Check sheet for the drawn part. Datum: minimum x, y, z corner. Units: mm. A direction names the side the tool comes from. Coordinates: 2 decimals unless noted, no trailing zeros. Loops run counter-clockwise (first coordinate to the right, second up) from the corner with the lowest first, then second, coordinate; pieces in that order, holes last.
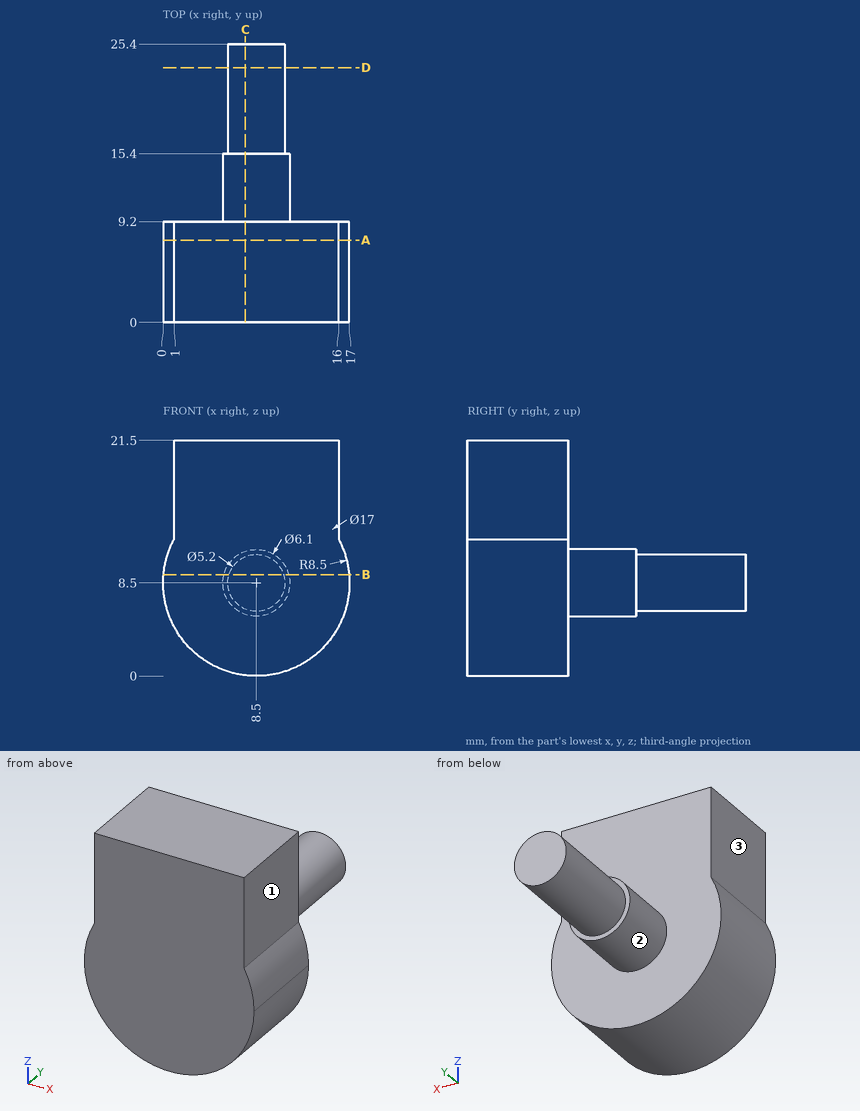
1) Scan lines: line 1 (X direction, y = 5.75, z = 16.75); line 2 (Y direction, x = 12, z = 16); line 3 (Z direction, x = 8.5, y = 11.75). Record each from-to range of solid material in increasing order.
Answer sheet:
line 1: x = 1 to 16
line 2: y = 0 to 9.2
line 3: z = 5.45 to 11.55
2) Depth check by flat-ended pin: pin 1 (4 mm diameter, centred on x = 9, y = 14.5, fed in from -Z); pin 2 (7 mm diameter, centred on y = 4, z = 16.5, fed in from +X); pin 3 (3 mm diameter, centred on y = 8, z = 15, fed in from -X); pin 4 (1 mm diameter, centred on y = 11.5, z = 19, fed in from +X). Enter the tip coordinate at first touch or a pass-through.
Answer sheet:
pin 1: stops at z = 5.45
pin 2: stops at x = 16
pin 3: stops at x = 1
pin 4: passes through
3) Section check D-D on y = 23.25. Enter the section's corners in (x, z), plus the area to 3 significant figures.
Answer sheet:
outline: circle Ø5.2 at (8.5, 8.5)
area: 21.2 mm2
4) Section check B-B on z = 9.25. Enter the section's corners in (x, y).
Answer sheet:
outline: (0.03, 0) - (16.97, 0) - (16.97, 9.2) - (11.46, 9.2) - (11.46, 15.4) - (10.99, 15.4) - (10.99, 25.4) - (6.01, 25.4) - (6.01, 15.4) - (5.54, 15.4) - (5.54, 9.2) - (0.03, 9.2) - close
5) Set-up check for the marked faces 1, 2 and 3: record each of +Z, -Z, +X, -X, +Y, -Y from which the full face is reachable in a straight line by a thin tool's end or side.
Answer sheet:
face 1: +Z, +X, +Y, -Y
face 2: +Y
face 3: +Z, -X, +Y, -Y
6) Section check A-A on y = 7.5. Enter the section's corners in (x, z).
Answer sheet:
outline: (1, 12.5) arc R8.5 ccw (long way) to (16, 12.5) - (16, 21.5) - (1, 21.5) - close
7) Section check C-C on x = 7.5. Enter the section's corners in (y, z), plus the area to 3 significant figures.
Answer sheet:
outline: (0, 0.06) - (9.2, 0.06) - (9.2, 5.62) - (15.4, 5.62) - (15.4, 6.1) - (25.4, 6.1) - (25.4, 10.9) - (15.4, 10.9) - (15.4, 11.38) - (9.2, 11.38) - (9.2, 21.5) - (0, 21.5) - close
area: 281 mm2
